```python
from build123d import *

# Parameters (mm, degrees)
F0_W     = 203.2
F0_H     = 406.4
F1_DEPTH = 50.8
F2_W     = 50.8
F2_H     = 254
F2_H_2   = 76.2
F3_DEPTH = 50.801


with BuildPart() as f1:
    # F0 (on Top) → F1 (new body)
    with BuildSketch(Plane.XY):
        Rectangle(F0_W, F0_H)
    extrude(amount=F1_DEPTH)

    # F2 (on face) → F3 (cut, through all)
    with BuildSketch(Plane.XY.offset(50.8)):
        Rectangle(F2_W, F2_H)
        with Locations((-76.2, -76.2)):
            Rectangle(F2_W, F2_H_2)
        with Locations((76.2, -76.2)):
            Rectangle(F2_W, F2_H_2)
    extrude(amount=-F3_DEPTH, mode=Mode.SUBTRACT)


solid = f1.part
```
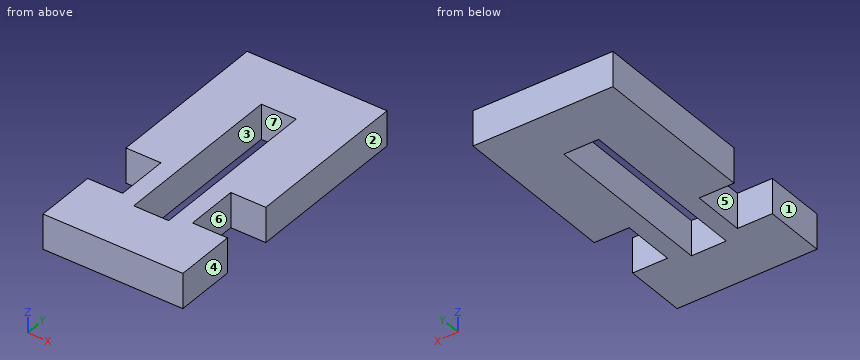
Build history of the part. All positions in model axes, mm. Face numbers are marked on the shaded views. A direction names the side the tool comes from. Give positions to 0.01 mm unless a question says otherwise; leave off trailing zeros. Order: outer loops, then holes, each group sorted by start corner. A loop starts at its lowest first (then second) coordinate and runs counter-clockwise, first axis right, second up. Notation, with made-up numbers: M 69,-16.5 L 83,-16.5 A29 cw 83,22.5 Z; hole C 86.5,-11.75 d10. An arc over 180 degrees is marked long. Write item = value, one per line. Start each with the question number.
(1) Probe L1, parallel to Y at x = -68, z = 42.5; L2, parallel to Y at x = -10, z = 41; L3, parallel to X at y = 86, z = 25.5. List the from-to ranges inside material, lowest first. Write a range as [from, to].
(2) Slice it at B-B on y = -6. Write the cut outline in (x, z), plus the area to 3 significant figures.
(3) Two-plate mould, pull along X, no slides. Class the marked faces 1, 2 and 3: released by +X, released by -X, zero draft, split by the parting line, or undercut.
(4) Slice it at A-A on x = 76. Write the cut outline in (y, z), plus the area to 3 significant figures.
(5) Pin check, flat tips, straight feed: pin 1 Ø8 at (x, y) = (29, 15.5) entering from -Z; pin 2 Ø15 at (y, z) = (-59.5, 27) entering from +X. Stop position of each tip, or through.
(6) Which spindle directions (+Z, -Z, +X, -X, +Y, -Y) get a long thin tool onto all of the face, cutting with end or side? Do the marked faces 4, 5, 6 and 7. Say none if no direction does.
(7) Slice it at C-C on z = 35.5. Write the cut outline in (x, y).
Responses:
q1.L1 = [-203.2, -114.3], [-38.1, 203.2]
q1.L2 = [-203.2, -127], [127, 203.2]
q1.L3 = [-101.6, -25.4], [25.4, 101.6]
q2.outline = M -101.6,0 L -25.4,0 L -25.4,50.8 L -101.6,50.8 Z; M 25.4,0 L 101.6,0 L 101.6,50.8 L 25.4,50.8 Z
q2.area = 7,740 mm2
q3.face_1 = released by -X
q3.face_2 = released by +X
q3.face_3 = undercut
q4.outline = M -203.2,0 L -114.3,0 L -114.3,50.8 L -203.2,50.8 Z; M -38.1,0 L 203.2,0 L 203.2,50.8 L -38.1,50.8 Z
q4.area = 16,800 mm2
q5.pin_1 = 0
q5.pin_2 = 50.8
q6.face_4 = +Z, -Z, +X, +Y, -Y
q6.face_5 = +Z, -Z, -X
q6.face_6 = +Z, -Z, +X
q6.face_7 = +Z, -Z
q7.outline = M -101.6,-203.2 L 101.6,-203.2 L 101.6,-114.3 L 50.8,-114.3 L 50.8,-38.1 L 101.6,-38.1 L 101.6,203.2 L -101.6,203.2 L -101.6,-38.1 L -50.8,-38.1 L -50.8,-114.3 L -101.6,-114.3 Z; hole M -25.4,-127 L 25.4,-127 L 25.4,127 L -25.4,127 Z
